Read the model definition and answer for the solid it produces. Units are mm, in the model's axes. Face numbers are marked on the shaded views. A direction names the side the tool comes from. Give positions to 0.01 mm unless a question says otherwise; leave off trailing zeros. Order: outer loops, then holes, each group sorted by start corner. A loop starts at its lowest first (then second) coordinate and runs counter-clockwise, first axis right, second up. Notation, with made-up numbers: (58, 23) - (101, 23) arc R19 cw to (101, 50) - close; hole circle Ø6 at (24, -32). An arc over 180 degrees is marked (long way). Write item = value, one per line.
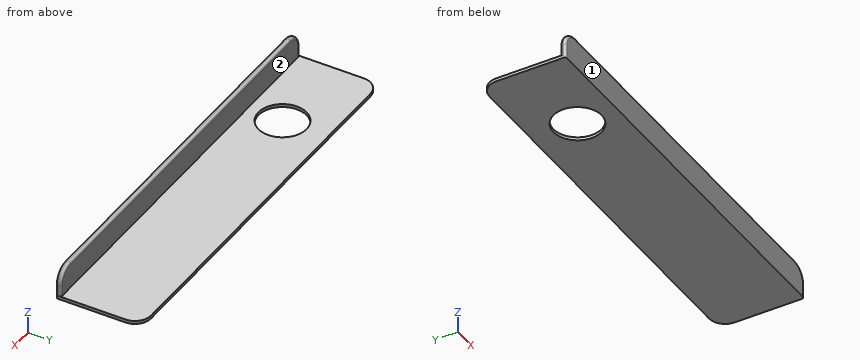
```python
from build123d import *

# Parameters (mm, degrees)
F1_DEPTH = 50.4
F2_R     = 3
F3_DEPTH = 0.401
F4_R     = 2
F5_R     = 0.3


with BuildPart() as f1:
    # F0 (on Right) → F1 (new body)
    with BuildSketch(Plane.YZ):
        Polygon((0, 3.8), (0, 0), (10.65, 0), (10.65, 0.4), (0.65, 0.4), (0.65, 3.8), align=None)
    extrude(amount=F1_DEPTH)

    # F2 (on face) → F3 (cut, through all)
    with BuildSketch(Plane.XY.offset(0.4)):
        with Locations((11, 5)):
            Circle(F2_R)
    extrude(amount=-F3_DEPTH, mode=Mode.SUBTRACT)

    # F4
    f4_edges = [f1.edges().sort_by_distance(p)[0] for p in [
        (0, 10.65, 0.2),
        (50.4, 10.65, 0.2),
        (50.4, 0.325, 3.8),
        (0, 0.325, 3.8),
    ]]
    fillet(f4_edges, radius=F4_R)

    # F5
    f5_edges = [f1.edges().sort_by_distance(p)[0] for p in [
        (0.585786, 0, 3.214214),
        (49.814214, 0, 3.214214),
        (50.4, 0.65, 1.1),
        (0, 0.65, 1.1),
    ]]
    fillet(f5_edges, radius=F5_R)


solid = f1.part
```
1. For the marked faces 1 and 2, determine the directions among +Z, -Z, +X, -X, +Y, -Y from which every point of the face is accessible in a straight line to the end or side of a thin tool.
Recorded:
face_1 = +Z, -Z, +X, -X, -Y
face_2 = +Z, +X, -X, +Y
2. Section D-D (x = 27) is taken. Determine the outline of the cut face in (y, z), and give its area (3 significant figures).
Recorded:
outline = (0, 0) - (10.65, 0) - (10.65, 0.4) - (0.65, 0.4) - (0.65, 3.5) arc R0.3 ccw to (0.35, 3.8) - (0.3, 3.8) arc R0.3 ccw to (0, 3.5) - close
area = 6.43 mm^2
3. Straight lines are drawn through the part: L1, parallel to Y at x = 11, z = 0.1; L2, parallel to Z at x = 16, y = 5.5; L3, parallel to Y at x = 39.5, z = 1.4. For each, find the intervals that lie inside material, in ascending order. Write a range as [from, to].
Recorded:
L1 = [0, 2], [8, 10.65]
L2 = [0, 0.4]
L3 = [0, 0.65]
4. Section B-B (y = 5) is taken. Determine the outline of the cut face in (x, z).
Recorded:
outline = (0, 0) - (8, 0) - (8, 0.4) - (0, 0.4) - close; (14, 0) - (50.4, 0) - (50.4, 0.4) - (14, 0.4) - close
5. Section A-A (x = 11) is taken. Determine the outline of the cut face in (y, z), and give its area (3 significant figures).
Recorded:
outline = (0, 0) - (2, 0) - (2, 0.4) - (0.65, 0.4) - (0.65, 3.5) arc R0.3 ccw to (0.35, 3.8) - (0.3, 3.8) arc R0.3 ccw to (0, 3.5) - close; (8, 0) - (10.65, 0) - (10.65, 0.4) - (8, 0.4) - close
area = 4.03 mm^2
6. Section C-C (z = 1.35) is taken. Determine the outline of the cut face in (x, y), and give its area (3 significant figures).
Recorded:
outline = (0, 0.3) arc R0.3 ccw to (0.3, 0) - (50.1, 0) arc R0.3 ccw to (50.4, 0.3) - (50.4, 0.35) arc R0.3 ccw to (50.1, 0.65) - (0.3, 0.65) arc R0.3 ccw to (0, 0.35) - close
area = 32.7 mm^2
